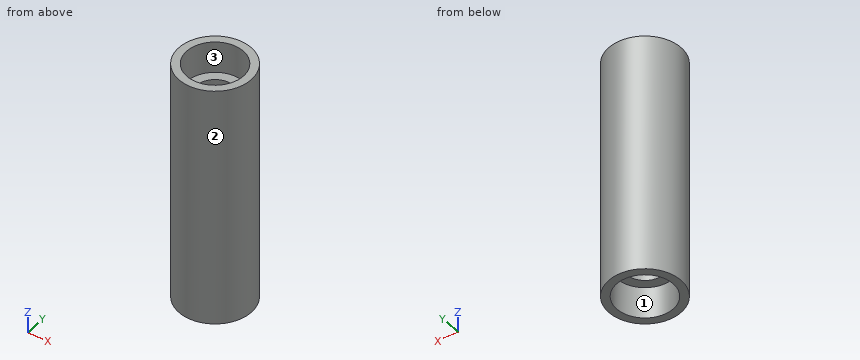
```python
from build123d import *

# Parameters (mm, degrees)
SKETCH2_R           = 5.75
SKETCH2_R_2         = 3
BOSS_EXTRUDE1_DEPTH = 19.2
SKETCH5_W           = 5
SKETCH5_H           = 4.5


with BuildPart() as part:
    # Sketch2 → Boss-Extrude1 (new, symmetric)
    with BuildSketch(Plane.XY):
        Circle(SKETCH2_R)
        Circle(SKETCH2_R_2, mode=Mode.SUBTRACT)
    extrude(amount=BOSS_EXTRUDE1_DEPTH, both=True)

    # Sketch5 → Cut-Revolve1 (revolve, cut)
    with BuildSketch(Plane(origin=(0, 0, 0), x_dir=(0, 0, -1), z_dir=(1, 0, 0)), mode=Mode.PRIVATE) as cut_revolve1_sk:
        with Locations((16.7, 2.25)):
            Rectangle(SKETCH5_W, SKETCH5_H)
        with Locations((-16.7, 2.25)):
            Rectangle(SKETCH5_W, SKETCH5_H)
    revolve(cut_revolve1_sk.sketch.rotate(Axis((0, 0, -19.2), (0, 0, 1)), 90), axis=Axis((0, 0, -19.2), (0, 0, 1)), mode=Mode.SUBTRACT)


solid = part.part
```
The model under review builds one solid part; all positions refer to its coordinate system, in mm. Face numbers are marked on the shaded views. Round coordinates to 2 decimals unless told otherwise and drop trailing zeros. Loops run counter-clockwise (first coordinate to the right, second up) from the corner with the lowest first, then second, coordinate; pieces in that order, holes last.
1) Wall thickness on line 1 along Y through (x, z) = (0, 0.25); line 2 along Z through (x, y) = (2.5, -3.5); line 3 along X through (y, z) = (-2, 5): over which ranges is each line inside the solid? List them lowest first.
Values follow:
line 1: y = -5.75 to -3, 3 to 5.75
line 2: z = -14.2 to 14.2
line 3: x = -5.39 to -2.24, 2.24 to 5.39
2) Consider section A-A on x = 0. State the section outline as (y, z) points.
Values follow:
outline: (-5.75, -19.2) - (-4.5, -19.2) - (-4.5, -14.2) - (-3, -14.2) - (-3, 14.2) - (-4.5, 14.2) - (-4.5, 19.2) - (-5.75, 19.2) - close; (3, -14.2) - (4.5, -14.2) - (4.5, -19.2) - (5.75, -19.2) - (5.75, 19.2) - (4.5, 19.2) - (4.5, 14.2) - (3, 14.2) - close
3) Consider section D-D on y = 5. State the section outline as (x, z) points, then the cut area to 3 significant figures.
Values follow:
outline: (-2.84, -19.2) - (2.84, -19.2) - (2.84, 19.2) - (-2.84, 19.2) - close
area: 218 mm2
4) Clearance check with flat-ended pins moving along their axes: P1, Ø1, axis at y = 4.5, z = -14, coming from the +X side; P2, Ø3, axis at y = 4.5, z = 12, coming from the -X side; P3, Ø5, axis at x = 0, y = 0, coming from the -Z side. State where each tip first meets the part, or that it passes through.
Values follow:
P1: stops at x = 4.13
P2: stops at x = -4.91
P3: passes through
5) Consider section C-C on z = -12.5. State the section outline as (x, y) points, then the cut area to 3 significant figures.
Values follow:
outline: circle Ø11.5 at (0, 0); hole circle Ø6 at (0, 0)
area: 75.6 mm2
6) The part is to be moulded in two halves that separate along Y. For the marked faces 1, 2 and 3, say which applies: pulls with the +Y half, pulls with the -Y half, needs draft (parallel to the pull), parting line crosses it, or undercut.
Values follow:
face 1: undercut
face 2: parting line crosses it
face 3: undercut
